The listing builds one solid part. Answer for the finished solid, in the listing's coordinates (mm). Face numbers are marked on the shaded views. A direction names the side the tool comes from. Round coordinates to 2 decimals unless told otherwise and drop trailing zeros. Loops run counter-clockwise (first coordinate to the right, second up) from the corner with the lowest first, then second, coordinate; pieces in that order, holes last. Notation, with made-up numbers: (-2, 14) - (29, 14) arc R25 ccw to (29, 37) - close; hole circle Ø6 at (32, -18.5). An arc over 180 degrees is marked (long way). One line per question, with ' | ' between items. Start each with the question number.
from build123d import *

# Parameters (mm, degrees)
F0_W          = 80
F0_H          = 40
F1_DEPTH      = 40
F1_DEPTH_BACK = 40
F2_W          = 76
F2_H          = 35
F3_DEPTH      = 78
F4_R          = 20.05
F5_DEPTH      = 3
F6_R          = 0.99999


# Not quite as in the source:
# - a fillet or chamfer is up to 0.001 mm smaller than in the source, because OpenCascade refuses the exact size


with BuildPart() as f1:
    # F0 (on Front) → F1 (new body, two sides)
    with BuildSketch(Plane.XZ) as f1_sk:
        Rectangle(F0_W, F0_H)
    extrude(amount=F1_DEPTH)
    extrude(f1_sk.sketch, amount=-F1_DEPTH_BACK)

    # F2 (on face) → F3 (cut)
    with BuildSketch(Plane.XZ.offset(40)):
        with Locations((0, -2.5)):
            Rectangle(F2_W, F2_H)
    extrude(amount=-F3_DEPTH, mode=Mode.SUBTRACT)

    # F4 (on face) → F5 (cut)
    with BuildSketch(Plane.XY.offset(20)):
        Circle(F4_R)
    extrude(amount=-F5_DEPTH, mode=Mode.SUBTRACT)

    # F6 (radius 1 in the source; OpenCascade refuses exactly that, so slightly less here)
    f6_edges = [f1.edges().sort_by_distance(p)[0] for p in [
        (40, -40, 0),
        (40, 0, 20),
        (40, 40, 0),
        (40, 0, -20),
        (-40, -40, 0),
        (0, -40, 20),
        (39, -40, -20),
        (38, -40, -2.5),
        (0, -40, 15),
        (-38, -40, -2.5),
        (-39, -40, -20),
        (-40, 0, 20),
        (0, 40, 20),
        (-20.05, 0, 20),
        (0, 40, -20),
        (-40, 40, 0),
        (-40, 0, -20),
    ]]
    fillet(f6_edges, radius=F6_R)


solid = f1.part
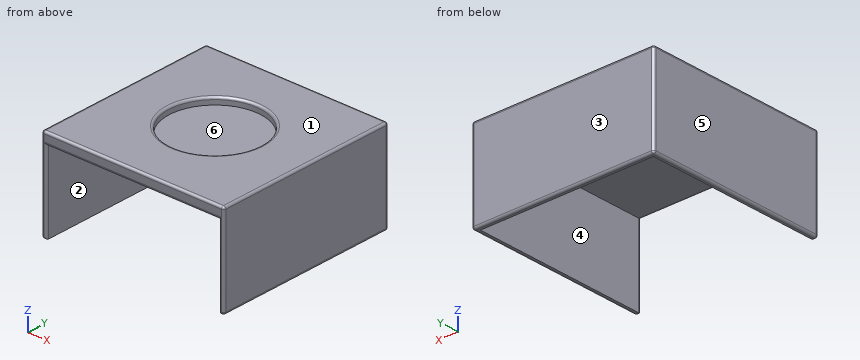
(1) Determine the mould class of the marked faces 3, 4, 5 and 6 for opening direction X: pulls with the +X half, pulls with the -X half, needs draft (parallel to the pull), parting line crosses it, or undercut.
(2) A tool of negligible diameter and unlimited length cuts with its end or side. For the marked faces 1 and 2, from which of +Z, -Z, +X, -X, +Y, -Y can it reach the whole face along a straight path? Write none if from no direction.
(3) Find section D-D on x = 0. Write down the section's boundary in (y, z), plus the area to 3 significant figures.
(4) Each of these flat-tipped pins is pushed along its axis until it touches: P1, Ø6, axis at x = -11, y = 0.5, coming from the +Z side; P2, Ø12, axis at x = -22, z = -3, coming from the -Y side; P3, Ø1.5, axis at x = -19, y = 9.5, coming from the -Z side. Where does it stop, or does it pass through?
(5) Consider L1, parallel to X at y = 15, z = -3.5; L2, parallel to Y at x = 0, z = 18.2; L3, parallel to Y at x = -34.5, z = -11. Determine where each line is inside the solid, lowest interval first.
(6) Find section A-A on x = 27.5. Write down the section's boundary in (y, z), plus the area to 3 significant figures.
(7) Find section C-C on y = 0. Write down the section's boundary in (x, z), plus the area to 3 significant figures.
Answer below:
1) face 3: needs draft | face 4: undercut | face 5: pulls with the -X half | face 6: undercut
2) face 1: +Z, +X, -X, +Y, -Y | face 2: -Z, -Y
3) outline: (-40, 16) arc R1 ccw to (-39, 15) - (38, 15) - (38, -20) - (39, -20) arc R1 ccw to (40, -19) - (40, 19) arc R1 ccw to (39, 20) - (21.05, 20) arc R1 ccw to (20.05, 19) - (20.05, 17) - (-20.05, 17) - (-20.05, 19) arc R1 ccw to (-21.05, 20) - (-39, 20) arc R1 ccw to (-40, 19) - close | area: 348 mm2
4) P1: z = 17 | P2: y = 38 | P3: z = 15
5) L1: -40 to -38, 38 to 40 | L2: -40 to -20.05, 20.05 to 40 | L3: 38 to 40
6) outline: (-40, 16) arc R1 ccw to (-39, 15) - (38, 15) - (38, -20) - (39, -20) arc R1 ccw to (40, -19) - (40, 19) arc R1 ccw to (39, 20) - (-39, 20) arc R1 ccw to (-40, 19) - close | area: 469 mm2
7) outline: (-40, -19) arc R1 ccw to (-39, -20) - (-38, -20) - (-38, 15) - (38, 15) - (38, -20) - (39, -20) arc R1 ccw to (40, -19) - (40, 19) arc R1 ccw to (39, 20) - (21.05, 20) arc R1 ccw to (20.05, 19) - (20.05, 17) - (-20.05, 17) - (-20.05, 19) arc R1 ccw to (-21.05, 20) - (-39, 20) arc R1 ccw to (-40, 19) - close | area: 418 mm2
